Model file for the job. Use its own axes, mm. Face numbers are marked on the shaded views. A direction names the side the tool comes from. Give positions to 0.01 mm unless a question says otherwise; leave off trailing zeros. Loops run counter-clockwise (first coordinate to the right, second up) from the corner with the lowest first, then second, coordinate; pieces in that order, holes last. Notation, with made-up numbers: (47.25, 18.5) - (78.25, 18.5) arc R35 ccw to (78.25, 51.5) - close; hole circle Ø8 at (84.5, 85). An arc over 180 degrees is marked (long way). Answer as CSV lines item,"result". Start each with the question number.
Item 1: Pin check, flat tips, straight feed: pin 1 (5 mm diameter, centred on x = 8.5, y = 5.5, fed in from +Z); pin 2 (0.9 mm diameter, centred on y = 0, z = 9.5, fed in from +X); pin 3 (1 mm diameter, centred on x = -0.5, z = 8.5, fed in from +Y); pin 4 (1 mm diameter, centred on x = 18.5, y = 0.5, fed in from +Z). Stop position of each tip, or through.
Item 2: Drill centre lines: L1, parallel to Y at x = 17.5, z = -1.75; L2, parallel to Z at x = 3, y = -3.5; L3, parallel to X at y = -1, z = 1. Where is each one in solid material? Low to high. Write a range as from..to.
Item 3: Saw through at D-D on y = -4.5. Give the cut face in (x, z).
Item 4: Pull direction Y, two halves, no side cores. Call the marked faces 4, 5 and 6: pulls with the +Y half, pulls with the -Y half, needs draft (parallel to the pull), parting line crosses it, or undercut.
Item 5: Saw through at A-A on x = 17.5. Give the cut face in (y, z).
Item 6: Saw through at C-C on x = 4. Give the cut face in (y, z).
Item 7: Tool access for the marked faces 1, 2 and 3: list every direction of +Z, -Z, +X, -X, +Y, -Y with a clear straight run to the whole face (end or side of a thin tool).
Item 8: Saw through at B-B on z = 2.5. Give the cut face in (x, y), plus the area to 3 significant figures.
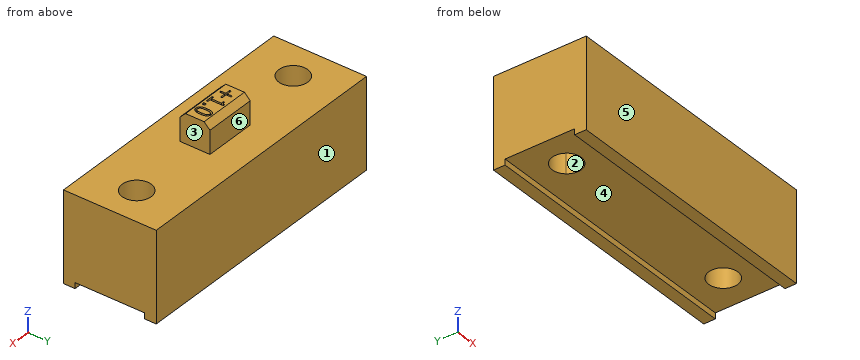
Autodesk Inventor part; units mm, degrees
ref_plane "YZ Plane" through (0, 0, 0) normal (1, 0, 0) x (0, 1, 0)
ref_plane "XZ Plane" through (0, 0, 0) normal (0, 1, 0) x (-1, 0, 0)
ref_plane "XY Plane" through (0, 0, 0) normal (0, 0, 1) x (1, 0, 0)
ref_plane "작업 평면1" through (23.5, -8, -2) normal (1, 0, 0) x (0, 0, -1)
sketch "스케치1" plane through (23.5, -8, -2) normal (1, 0, 0) x (0, 0, -1)
  line L0 (0, 16) -> (-8.15, 16)
  line L1 (-8.15, 16) -> (-8.15, 10.6)
  line L2 (-8.15, 10.6) -> (-12.15, 10.6)
  line L3 (-13.15, 9.6) -> (-12.15, 10.6)
  line L4 (-13.15, 9.6) -> (-13.15, 6.4)
  line L5 (-12.15, 5.4) -> (-13.15, 6.4)
  line L6 (-12.15, 5.4) -> (-8.15, 5.4)
  line L7 (-8.15, 5.4) -> (-8.15, 0)
  line L8 (-8.15, 0) -> (0, 0)
  line L9 (0, 16) -> (7.35, 16)
  line L10 (7.35, 16) -> (7.35, 15)
  line L11 (0, 0) -> (7.35, 0)
  line L12 (7.35, 0) -> (7.35, 1)
  line L13 (0, 16) -> (-8.15, 16)
  line L14 (-8.15, 10.6) -> (-12.15, 10.6)
  line L15 (-8.15, 10.6) -> (-12.15, 10.6)
  line L16 (-12.15, 10.6) -> (-13.15, 9.6)
  line L17 (-13.15, 6.4) -> (-12.15, 5.4)
  line L18 (6.35, 14) -> (7.35, 14)
  line L19 (7.35, 14) -> (7.35, 15)
  line L20 (6.35, 2) -> (7.35, 2)
  line L21 (7.35, 2) -> (7.35, 1)
  line L22 (6.35, 14) -> (6.35, 2)
  point P0 (-2, 8)
  point P1 (4.35, 10.6)
  point P2 (4.35, 5.4)
  dimension "d1" = 7.35
  dimension "d13" = 7.35
sketch "스케치2" plane through (-23.5, 8, 6.15) normal (0, 0, 1) x (1, 0, 0)
  arc A0 (7.9209, -9.6) -> (7.9209, -6.4) centre (6, -8) ccw
  line L0 (39.0791, -9.6) -> (7.9209, -9.6)
  circle A1 centre (6, -8) radius 2.5
  circle A2 centre (41, -8) radius 2.5
  circle A3 centre (41, -8) radius 2.5
  point P0 (23.5, -8)
  point P1 (7.9209, -6.4)
extrude "돌출1" add sketch "스케치1" against normal up to surface (47 mm away)
extrude "돌출2" cut sketch "스케치2" along normal mid plane 50
sketch "스케치3" plane through (-15.5791, 1.6, 11.15) normal (0, 0, 1) x (1, 0, 0)
  line L0 (15.5791, -14.4593) -> (15.5791, 15.5737)
  line L1 (-7.9209, 4.4) -> (-7.9209, -7.6)
  line L2 (-7.9209, 4.4) -> (11.0791, 4.4)
  line L3 (11.0791, 4.4) -> (11.0791, -7.6)
  line L4 (11.0791, -7.6) -> (-7.9209, -7.6)
  line L5 (-7.9209, -7.6) -> (-7.9209, 4.4)
  line L6 (39.0791, 4.4) -> (39.0791, -7.6)
  line L7 (39.0791, 4.4) -> (20.0791, 4.4)
  line L8 (20.0791, 4.4) -> (20.0791, -7.6)
  line L9 (20.0791, -7.6) -> (39.0791, -7.6)
  line L10 (39.0791, -7.6) -> (39.0791, 4.4)
  point P0 (15.5791, -1.6)
  dimension "d9" = 19
extrude "돌출3" cut sketch "스케치3" against normal up to surface (5 mm away)
sketch "스케치4" plane through (-4.5, 1.6, 11.15) normal (0, 0, 1) x (1, 0, 0)
  line L0 (0.6181, -0.2528) -> (7.2489, -0.2528) construction
  line L1 (7.2489, -0.2528) -> (7.2489, -2.6222) construction
  line L2 (7.2489, -2.6222) -> (0.6181, -2.6222) construction
  line L3 (0.6181, -2.6222) -> (0.6181, -0.2528) construction
  line L4 (2.8925, -1.8686) -> (2.0321, -1.8686)
  line L5 (2.0321, -1.8686) -> (2.0321, -2.729)
  line L6 (2.0321, -2.729) -> (1.7481, -2.729)
  line L7 (1.7481, -2.729) -> (1.7481, -1.8686)
  line L8 (1.7481, -1.8686) -> (0.8877, -1.8686)
  line L9 (0.8877, -1.8686) -> (0.8877, -1.5949)
  line L10 (0.8877, -1.5949) -> (1.7481, -1.5949)
  line L11 (1.7481, -1.5949) -> (1.7481, -0.7345)
  line L12 (1.7481, -0.7345) -> (2.0321, -0.7345)
  line L13 (2.0321, -0.7345) -> (2.0321, -1.5949)
  line L14 (2.0321, -1.5949) -> (2.8925, -1.5949)
  line L15 (2.8925, -1.5949) -> (2.8925, -1.8686)
  line L16 (4.7842, -2.8443) -> (3.545, -2.8443)
  line L17 (3.545, -2.8443) -> (3.545, -2.5849)
  line L18 (3.545, -2.5849) -> (4.0061, -2.5849)
  line L19 (4.0061, -2.5849) -> (4.0061, -0.8827)
  line L20 (4.0061, -0.8827) -> (3.545, -0.8827)
  line L21 (3.545, -0.8827) -> (3.545, -0.6501)
  spline S0 degree 2 poles (3.545, -0.6501) (3.8064, -0.6501) (4.0534, -0.5019) (4.0699, -0.2961) knots 0 0 0 1 2 2 2
  line L22 (4.0699, -0.2961) -> (4.3334, -0.2961)
  line L23 (4.3334, -0.2961) -> (4.3334, -2.5849)
  line L24 (4.3334, -2.5849) -> (4.7842, -2.5849)
  line L25 (4.7842, -2.5849) -> (4.7842, -2.8443)
  line L26 (5.7969, -2.8443) -> (5.3893, -2.8443)
  line L27 (5.3893, -2.8443) -> (5.3893, -2.3585)
  line L28 (5.3893, -2.3585) -> (5.7969, -2.3585)
  line L29 (5.7969, -2.3585) -> (5.7969, -2.8443)
  spline S1 degree 2 poles (7.8902, -1.5743) (7.8902, -2.2577) (7.4929, -2.8978) (7.0792, -2.8978) knots 0 0 0 1 2 2 2
  spline S2 degree 2 poles (7.0792, -2.8978) (6.6593, -2.8978) (6.2662, -2.2453) (6.2662, -1.5763) knots 0 0 0 1 2 2 2
  spline S3 degree 2 poles (6.2662, -1.5763) (6.2662, -0.8889) (6.6634, -0.2528) (7.0792, -0.2528) knots 0 0 0 1 2 2 2
  spline S4 degree 2 poles (7.0792, -0.2528) (7.4971, -0.2528) (7.8902, -0.9115) (7.8902, -1.5743) knots 0 0 0 1 2 2 2
  spline S5 degree 2 poles (7.4538, -2.3482) (7.5032, -2.2227) (7.5444, -1.8357) (7.5444, -1.5743) knots 0 0 0 1 2 2 2
  spline S6 degree 2 poles (7.5444, -1.5743) (7.5444, -1.3129) (7.5032, -0.928) (7.4518, -0.7983) knots 0 0 0 1 2 2 2
  spline S7 degree 2 poles (7.4518, -0.7983) (7.4003, -0.6686) (7.2212, -0.5348) (7.0792, -0.5348) knots 0 0 0 1 2 2 2
  spline S8 degree 2 poles (7.0792, -0.5348) (6.9372, -0.5348) (6.754, -0.6686) (6.7005, -0.8024) knots 0 0 0 1 2 2 2
  spline S9 degree 2 poles (6.7005, -0.8024) (6.649, -0.9321) (6.612, -1.3273) (6.612, -1.5763) knots 0 0 0 1 2 2 2
  spline S10 degree 2 poles (6.612, -1.5763) (6.612, -1.8439) (6.6449, -2.2021) (6.6984, -2.342) knots 0 0 0 1 2 2 2
  spline S11 degree 2 poles (6.6984, -2.342) (6.7478, -2.4738) (6.931, -2.6158) (7.0792, -2.6158) knots 0 0 0 1 2 2 2
  spline S12 degree 2 poles (7.0792, -2.6158) (7.2192, -2.6158) (7.4024, -2.482) (7.4538, -2.3482) knots 0 0 0 1 2 2 2
  point P0 (4.5, -1.6)
extrude "돌출4" cut sketch "스케치4" against normal blind 5
properties part number "Bearing Spacer_V2_1mm"
Responses:
1,pin 1,"z = 6.15"
1,pin 2,"x = 4.5"
1,pin 3,"y = 2.6"
1,pin 4,"through"
2,L1,"-8..-2.5, 2.5..8"
2,L2,"-8.35..6.15"
2,L3,"-23.5..-19.79, -15.21..15.21, 19.79..23.5"
3,outline,"(-23.5, -8.35) - (23.5, -8.35) - (23.5, 6.15) - (-23.5, 6.15) - close"
4,face 4,"undercut"
4,face 5,"pulls with the -Y half"
4,face 6,"pulls with the +Y half"
5,outline,"(-8, -9.35) - (-6, -9.35) - (-6, -8.35) - (-2.5, -8.35) - (-2.5, 6.15) - (-8, 6.15) - close; (2.5, -8.35) - (6, -8.35) - (6, -9.35) - (8, -9.35) - (8, 6.15) - (2.5, 6.15) - close"
6,outline,"(-8, -9.35) - (-6, -9.35) - (-6, -8.35) - (6, -8.35) - (6, -9.35) - (8, -9.35) - (8, 6.15) - (2.6, 6.15) - (2.6, 10.15) - (1.6, 11.15) - (-1.6, 11.15) - (-2.6, 10.15) - (-2.6, 6.15) - (-8, 6.15) - close"
7,face 1,"+Z, -Z, +X, -X, +Y"
7,face 2,"+Z, -Z"
7,face 3,"+Z, +X, +Y, -Y"
8,outline,"(-23.5, -8) - (23.5, -8) - (23.5, 8) - (-23.5, 8) - close; hole circle Ø5 at (-17.5, 0); hole circle Ø5 at (17.5, 0)"
8,area,"713 mm2"
